Part model, mm, in its own coordinate system. A direction names the side the tool comes from. Coordinates: 2 decimals unless noted, no trailing zeros. Loops run counter-clockwise (first coordinate to the right, second up) from the corner with the lowest first, then second, coordinate; pieces in that order, holes last. Notation, with made-up numbers: (86.5, 86) - (105.5, 86) arc R15 ccw to (105.5, 103) - close; hole circle Ø11 at (64, 72.5). An arc over 180 degrees is marked (long way). Answer as CSV lines item,"result".
from build123d import *

# Parameters (mm, degrees)
BOSS_EXTRUDE1_DEPTH = 30
CUT_EXTRUDE1_DEPTH  = 60
SKETCH6_R           = 5
BOSS_EXTRUDE2_DEPTH = 36


with BuildPart() as part:
    # Sketch4 → Boss-Extrude1 (new body, symmetric)
    with BuildSketch(Plane(origin=(0, 0, 0), x_dir=(0, 0, -1), z_dir=(1, 0, 0))):
        with BuildLine():
            Line((-7.5, 90), (7.5, 90))
            Line((7.5, 90), (7.5, 34))
            ThreePointArc((7.5, 34), (13.357864376, 19.857864376), (27.5, 14))
            Line((27.5, 14), (47.5, 14))
            Line((47.5, 14), (47.5, 0))
            Line((47.5, 0), (7.5, 0))
            Line((7.5, 0), (7.5, 6))
            Line((7.5, 6), (-7.5, 6))
            Line((-7.5, 6), (-7.5, 0))
            Line((-7.5, 0), (-47.5, 0))
            Line((-47.5, 0), (-47.5, 14))
            Line((-47.5, 14), (-27.5, 14))
            ThreePointArc((-27.5, 14), (-13.357864376, 19.857864376), (-7.5, 34))
            Line((-7.5, 34), (-7.5, 90))
        make_face()
    extrude(amount=BOSS_EXTRUDE1_DEPTH, both=True)

    # Sketch5 → Cut-Extrude1 (cut)
    with BuildSketch(Plane.XY.offset(7.5)):
        with BuildLine():
            Line((8, 70), (8, 90))
            Line((8, 90), (-8, 90))
            Line((-8, 90), (-8, 70))
            ThreePointArc((-8, 70), (0, 62), (8, 70))
        make_face()
    extrude(amount=-CUT_EXTRUDE1_DEPTH, mode=Mode.SUBTRACT)

    # Sketch6 → Boss-Extrude2 (add)
    with BuildSketch(Plane(origin=(0, 50, 0), x_dir=(1, 0, 0), z_dir=(0, 1, 0))):
        with BuildLine():
            Line((-10, -23.46544552), (-10, -7.5))
            Line((-10, -7.5), (10, -7.5))
            Line((10, -7.5), (10, -23.46544552))
            ThreePointArc((10, -23.46544552), (0, -33.46544552), (-10, -23.46544552))
        make_face()
        with Locations((0, -23.46544552)):
            Circle(SKETCH6_R, mode=Mode.SUBTRACT)
    extrude(amount=-BOSS_EXTRUDE2_DEPTH)


solid = part.part
Q1. Saw through at A-A (y = 44). Give the cut face in (x, z).
Results:
outline,"(-30, -7.5) - (30, -7.5) - (30, 7.5) - (10, 7.5) - (10, 23.47) arc R10 ccw to (-10, 23.47) - (-10, 7.5) - (-30, 7.5) - close; hole circle Ø10 at (0, 23.47)"
Q2. Flat gauge pins, fed straight in: pin 1 (22 mm diameter, centred on x = -13, z = -42.5, fed in from +Y); pin 2 (10 mm diameter, centred on y = 65, z = -13.5, fed in from -X); pin 3 (10 mm diameter, centred on x = -12, y = 33.5, fed in from -Z); pin 4 (11.5 mm diameter, centred on x = 0, z = 23.47, fed in from +Y). Where does each tip first touch, or does it go through?
Results:
pin 1,"stops at y = 14"
pin 2,"passes through"
pin 3,"stops at z = -8.27"
pin 4,"stops at y = 50"
Q3. Saw through at B-B (y = 74). Give the cut face in (x, z).
Results:
outline,"(-30, -7.5) - (-8, -7.5) - (-8, 7.5) - (-30, 7.5) - close; (8, -7.5) - (30, -7.5) - (30, 7.5) - (8, 7.5) - close"
Q4. Which spindle directions (+Z, -Z, +X, -X, +Y, -Y) get a long thin tool onto all of the face, cutting with end or side? Do faces 5 (the face through (0.22, 32.252, 33.463)), 6 (the face through (-10, 32, 16)), 7 (the face through (0.06, 14.53, 22.92)), 8 (the face through (0, 6, 0)). Say none if no direction does.
Results:
face 5,"+Z, +Y"
face 6,"+Z, -X, +Y"
face 7,"+Y"
face 8,"+X, -X, -Y"
Q5. Two-plate mould, pull along Z, no slides. Class faces 1 (the face through (19.721, 19.703, 13.514)), 2 (the face through (0, 7, -47.5)), 3 (the face through (-1.084, 32.252, 28.347)), 4 (the face through (0, 3, 7.5)): released by +Z, released by -Z, zero draft, split by the parting line, or undercut.
Results:
face 1,"released by +Z"
face 2,"released by -Z"
face 3,"undercut"
face 4,"undercut"
Q6. Saw through at D-D (z = -29). Give the cut face in (x, y).
Results:
outline,"(-30, 0) - (30, 0) - (30, 14) - (-30, 14) - close"
Q7. Wall check: L1, parallel to X at y = 82, z = 3; L2, parallel to Y at x = -22, z = -4; L3, parallel to Z at x = 0, y = 40. Give the ranges that are in metal, low to high.
Results:
L1,"x = -30 to -8, 8 to 30"
L2,"y = 6 to 90"
L3,"z = -7.5 to 18.47, 28.47 to 33.47"
Q8. Saw through at C-C (x = 19). Give the cut face in (y, z).
Results:
outline,"(0, -47.5) - (14, -47.5) - (14, -27.5) arc R20 cw to (34, -7.5) - (90, -7.5) - (90, 7.5) - (34, 7.5) arc R20 cw to (14, 27.5) - (14, 47.5) - (0, 47.5) - (0, 7.5) - (6, 7.5) - (6, -7.5) - (0, -7.5) - close"
